Check sheet for the modelled part. Datum: model origin and axes. Units: mm. Face numbers are marked on the shaded views. Coordinates: 2 decimals unless noted, no trailing zeros. Loops run counter-clockwise (first coordinate to the right, second up) from the corner with the lowest first, then second, coordinate; pieces in that order, holes last.
```python
from build123d import *

# Parameters (mm, degrees)
SKETCH1_W           = 63.5
SKETCH1_H           = 25.4
BOSS_EXTRUDE1_DEPTH = 6.35
SKETCH3_R           = 1.5875
CUT_EXTRUDE2_DEPTH  = 66.068137364
FILLET1_R           = 3.175
SKETCH4_R           = 4.7625
CUT_EXTRUDE3_DEPTH  = 38.701036126
SKETCH5_W           = 1.5875
SKETCH5_H           = 6.35
CUT_EXTRUDE4_DEPTH  = 3.175
SKETCH6_R           = 0.79375
BOSS_EXTRUDE2_DEPTH = 3.048


with BuildPart() as part:
    # Sketch1 → Boss-Extrude1 (new body)
    with BuildSketch(Plane.XY):
        with Locations((-3.175, 0)):
            Rectangle(SKETCH1_W, SKETCH1_H)
    extrude(amount=BOSS_EXTRUDE1_DEPTH)

    # Sketch3 → Cut-Extrude2 (cut, through all)
    with BuildSketch(Plane(origin=(28.575, 0, 6.35), x_dir=(0, 0, -1), z_dir=(1, 0, 0))):
        with Locations((3.175, -9.525)):
            Circle(SKETCH3_R)
    extrude(amount=-CUT_EXTRUDE2_DEPTH, mode=Mode.SUBTRACT)

    # Fillet1
    fillet1_edges = [part.edges().sort_by_distance(p)[0] for p in [
        (-3.175, -12.7, 0),
        (-3.175, -12.7, 6.35),
    ]]
    fillet(fillet1_edges, radius=FILLET1_R - 0.0001)  # a hair under: the kernel refuses the full size

    # Sketch4 → Cut-Extrude3 (cut, through all)
    with BuildSketch(Plane(origin=(0, 0, 0), x_dir=(-1, 0, 0), z_dir=(0, 0, -1))):
        with Locations((22.225, 3.175)):
            Circle(SKETCH4_R)
    extrude(amount=-CUT_EXTRUDE3_DEPTH, mode=Mode.SUBTRACT)

    # Sketch5 → Cut-Extrude4 (cut)
    with BuildSketch(Plane(origin=(28.575, 0, 0), x_dir=(0, 0, -1), z_dir=(1, 0, 0))):
        with Locations((-3.175, -7.9375)):
            Rectangle(SKETCH5_W, SKETCH5_H)
    extrude(amount=-CUT_EXTRUDE4_DEPTH, mode=Mode.SUBTRACT)

    # Sketch6 → Boss-Extrude2 (add)
    with BuildSketch(Plane(origin=(28.575, 0, 0), x_dir=(0, 0, -1), z_dir=(1, 0, 0))):
        with Locations(Location((-3.209540098, 0.635, 0), (0, 0, 180))):
            Circle(SKETCH6_R)
    extrude(amount=BOSS_EXTRUDE2_DEPTH)


solid = part.part
```
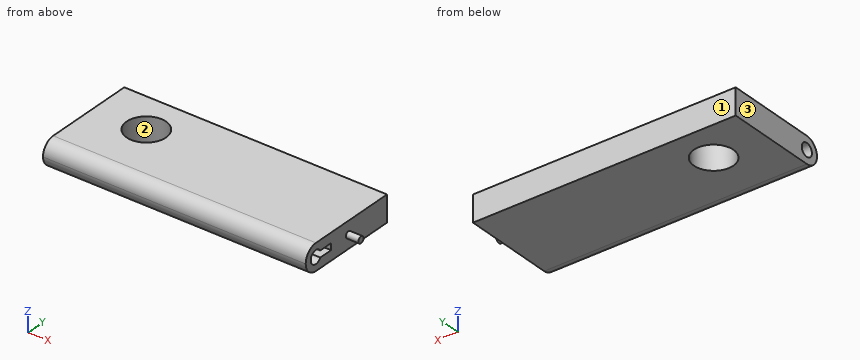
1) Section check B-B on y = 2.5. Enter the section's corners in (x, z) (3 decimals), plus the area to 3 significant figures.
Answer sheet:
outline: (-34.925, 0) - (-26.939, 0) - (-26.939, 6.35) - (-34.925, 6.35) - close; (-17.511, 0) - (28.575, 0) - (28.575, 6.35) - (-17.511, 6.35) - close
area: 343 mm2
2) Depth check by flat-ended pin: pin 1 (5.5 mm diameter, centred on x = -22.225, y = 3.175, fed in from -Z); pin 2 (1.7 mm diameter, centred on y = -6, z = 3, fed in from +X) (3 decimals). Enter the tip coordinate at first touch or a pass-through.
Answer sheet:
pin 1: passes through
pin 2: stops at x = 28.575
3) Section check C-C on x = -22. Give the number of separate pieces and of enclosed holes in the cut face, plus the area to 3 significant figures.
Answer sheet:
separate pieces: 2
enclosed holes: 1
area: 88.6 mm2
4) Mould release check, pull along X, two halves, no side actions. Record for the marked faces 1, 2 and 3: +X half, -X half, draft (parallel to the pull), parting line (faces both ways), or undercut.
Answer sheet:
face 1: draft
face 2: undercut
face 3: -X half
5) Scan lines: line 1 (Y direction, x = 23.5, z = 3); line 2 (Z direction, x = -5.5, y = -9.5); line 3 (X direction, y = 9, z = 0.5) (3 decimals). Record each from-to range of solid material in increasing order.
Answer sheet:
line 1: y = -12.7 to -11.1, -7.95 to 12.7
line 2: z = 0 to 1.59, 4.76 to 6.35
line 3: x = -34.925 to 28.575
6) Section check D-D on y = -6.75. Enter the section's corners in (x, z) (3 decimals), plus the area to 3 significant figures.
Answer sheet:
outline: (-34.925, 0) - (28.575, 0) - (28.575, 2.381) - (25.4, 2.381) - (25.4, 3.969) - (28.575, 3.969) - (28.575, 6.35) - (-34.925, 6.35) - close
area: 398 mm2
